Part print with two shaded views. Sizes in mm from the minimum x, y, z corner. A direction names the side the tool comes from. Round coordinates to 2 decimals unless told otherwise and drop trailing zeros. Order: outer loops, then holes, each group sorted by start corner. A loop starts at its lowest first (then second) coordinate and runs counter-clockwise, first axis right, second up. Notation, with made-up numbers: (72, 1.25) -> (90, 1.25) arc R15 cw to (90, 16.25) -> close; hole circle Ø8 at (51, 73.5). An arc over 180 degrees is marked (long way). Answer as a JSON object with one key per item and string values.
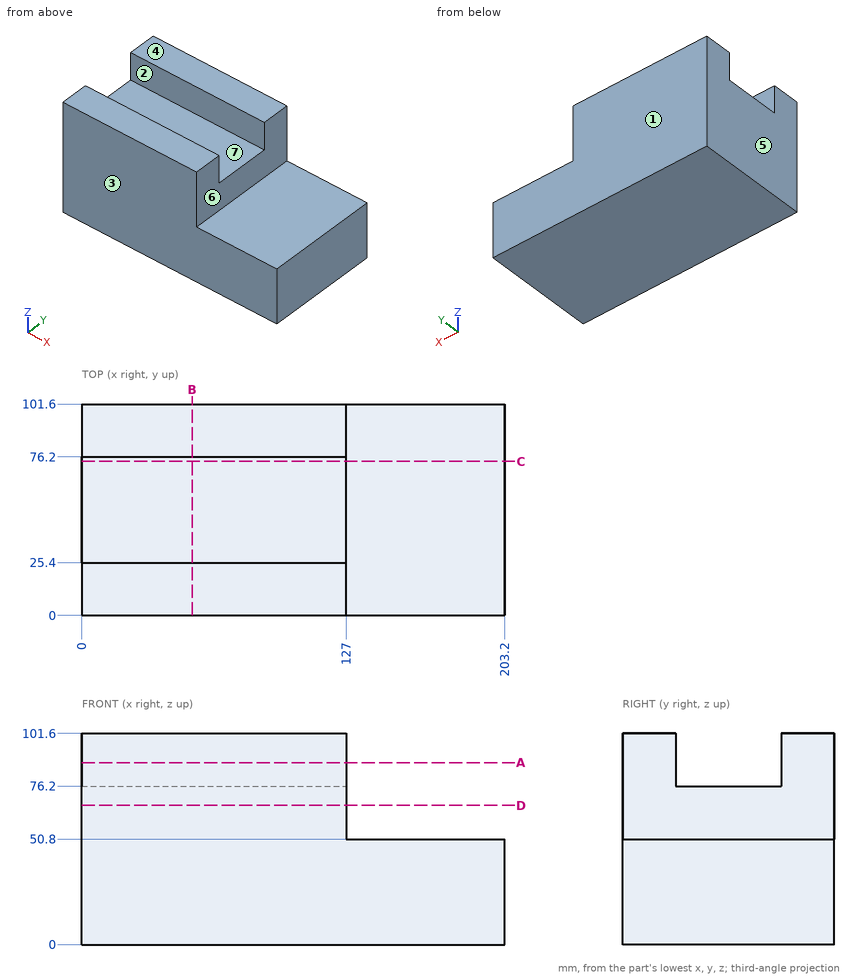
1) Which spindle directions (+Z, -Z, +X, -X, +Y, -Y) get a long thin tool onto all of the face, cutting with end or side? Do the marked faces 5, 6 and 7. Say none if no direction does.
Checked values:
{"face 5": "+Z, -Z, -X, +Y, -Y", "face 6": "+Z, +X, +Y, -Y", "face 7": "+Z, +X, -X"}
2) Flat gauge pins, fed straight in: pin 1 Ø5 at (x, y) = (76, 46) entering from +Z; pin 2 Ø1 at (x, y) = (138.5, 27) entering from +Z. Where does each tip first touch, or does it go through?
Checked values:
{"pin 1": "stops at z = 76.2", "pin 2": "stops at z = 50.8"}
3) Cut at C-C, the plane y = 74. Give the cut face in (x, z), plus the area to 3 significant figures.
Checked values:
{"outline": "(0, 0) -> (203.2, 0) -> (203.2, 50.8) -> (127, 50.8) -> (127, 76.2) -> (0, 76.2) -> close", "area": "13,500 mm²"}
4) Cut at A-A, the plane z = 87.5. Give the cut face in (x, y).
Checked values:
{"outline": "(0, 0) -> (127, 0) -> (127, 25.4) -> (0, 25.4) -> close; (0, 76.2) -> (127, 76.2) -> (127, 101.6) -> (0, 101.6) -> close"}
5) Probe L1, parallel to Y at x = 92, z = 85.5; L2, parallel to Z at x = 160.5, y = 38.5; L3, parallel to X at y = 89, z = 67.5. List the from-to ranges inside material, lowest first. Write a range as from..to.
Checked values:
{"L1": "y = 0..25.4, 76.2..101.6", "L2": "z = 0..50.8", "L3": "x = 0..127"}
6) Cut at D-D, the plane z = 67. Give the cut face in (x, y).
Checked values:
{"outline": "(0, 0) -> (127, 0) -> (127, 101.6) -> (0, 101.6) -> close"}
7) Pull direction Y, two halves, no side cores. Call the marked faces 1, 2, 3 and 4: pulls with the +Y half, pulls with the -Y half, needs draft (parallel to the pull), parting line crosses it, or undercut.
Checked values:
{"face 1": "pulls with the +Y half", "face 2": "undercut", "face 3": "pulls with the -Y half", "face 4": "needs draft"}
8) Cut at B-B, the plane x = 53. Give the cut face in (y, z).
Checked values:
{"outline": "(0, 0) -> (101.6, 0) -> (101.6, 101.6) -> (76.2, 101.6) -> (76.2, 76.2) -> (25.4, 76.2) -> (25.4, 101.6) -> (0, 101.6) -> close"}
